Design review of the part built by this model. Coordinates are the model's own, in mm. Face numbers are marked on the shaded views. A direction names the side the tool comes from. Give positions to 0.01 mm unless a question says otherwise; leave off trailing zeros. Order: outer loops, then holes, each group sorted by start corner. A loop starts at its lowest first (then second) coordinate and runs counter-clockwise, first axis right, second up.
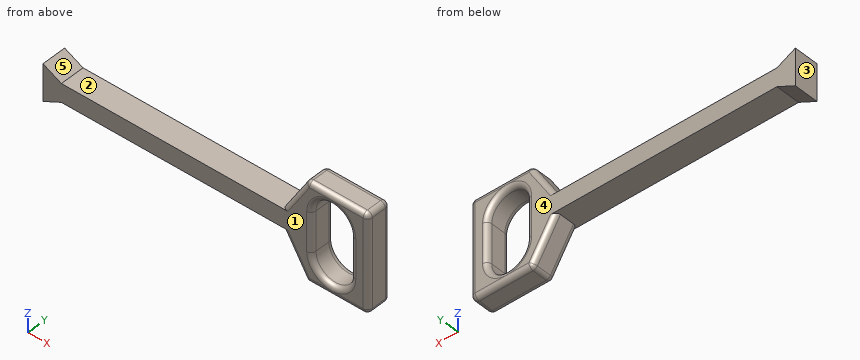
```python
from build123d import *

# Parameters (mm, degrees)
BOSS_EXTRUDE1_DEPTH = 10
FILLET1_R           = 2
FILLET2_R           = 2


with BuildPart() as part:
    # Sketch1 → Boss-Extrude1 (new body)
    with BuildSketch(Plane(origin=(0, 0, 0), x_dir=(1, 0, 0), z_dir=(0, 1, 0))):
        Polygon((0, 0), (0, -7.5), (7.5, -3.75), (97.5, -3.75), (107.5, -20), (132.5, -20), (132.5, 20), (107.5, 20), (97.5, 3.75), (7.5, 3.75), (0, 7.5), align=None)
        with BuildLine():
            Line((125.5, 8), (125.5, -8))
            ThreePointArc((125.5, -8), (117.5, -16), (109.5, -8))
            Line((109.5, -8), (109.5, 8))
            ThreePointArc((109.5, 8), (117.5, 16), (125.5, 8))
        make_face(mode=Mode.SUBTRACT)
    extrude(amount=BOSS_EXTRUDE1_DEPTH)

    # Fillet1
    fillet1_edges = [part.edges().sort_by_distance(p)[0] for p in [
        (117.5, 0, -16),
        (109.5, 0, 0),
        (117.5, 0, 16),
        (125.5, 0, 0),
        (117.5, 10, -16),
        (109.5, 10, 0),
        (117.5, 10, 16),
        (125.5, 10, 0),
    ]]
    fillet(fillet1_edges, radius=FILLET1_R)

    # Fillet2
    fillet2_edges = [part.edges().sort_by_distance(p)[0] for p in [
        (102.5, 0, -11.875),
        (120, 0, -20),
        (132.5, 0, 0),
        (120, 0, 20),
        (102.5, 0, 11.875),
        (102.5, 10, 11.875),
        (107.5, 5, -20),
        (132.5, 5, -20),
        (132.5, 5, 20),
        (107.5, 5, 20),
        (120, 10, 20),
        (132.5, 10, 0),
        (120, 10, -20),
        (102.5, 10, -11.875),
    ]]
    fillet(fillet2_edges, radius=FILLET2_R - 0.0001)  # a hair under: the kernel refuses the full size


solid = part.part
```
1. For pin 1 (3 mm diameter, centred on x = 69, y = 5.5, fed in from +Z); pin 2 (1.5 mm diameter, centred on y = 8.5, z = 12.5, fed in from -X); pin 3 (1 mm diameter, centred on y = 7, z = 12, fed in from -X), all flat-tipped, find the tip position at first contact; note any pin that passes through.
Recorded:
pin 1: stops at z = 3.75
pin 2: stops at x = 102.47
pin 3: stops at x = 102.27
2. Machinability: for the marked faces 4 and 5, which of the approach directions +Z, -Z, +X, -X, +Y, -Y give a long, thin tool a straight path to every point of the face, cutting with its end or side? Answer none if there is none.
Recorded:
face 4: +Z, -Z, +X, -X, +Y
face 5: +Z, +Y, -Y
3. Take a section at B-B (x = 73). State the section outline as (y, z) points.
Recorded:
outline: (0, -3.75) - (10, -3.75) - (10, 3.75) - (0, 3.75) - close
4. For line 1 along X through (y, z) = (6.5, 0); line 2 along Z through (x, y) = (85, 9.25), list the stretches that pass through material, from the lowest coordinate up.
Recorded:
line 1: x = 0 to 109.5, 125.5 to 132.5
line 2: z = -3.75 to 3.75
5. Draft analysis for pull direction X (two halves, no side actions). For the marked faces 1, 2 and 3, state which applies: pulls with the +X half, pulls with the -X half, needs draft (parallel to the pull), parting line crosses it, or undercut.
Recorded:
face 1: needs draft
face 2: undercut
face 3: pulls with the -X half
